from build123d import *

# Parameters (mm, degrees)
F0_R     = 12.7
F1_DEPTH = 152.4
F3_DEPTH = 127
F4_R     = 25.4
F5_SIZE  = 12.7


with BuildPart() as f1:
    # F0 (on Top) → F1 (new body)
    with BuildSketch(Plane.XY):
        with BuildLine():
            Line((127, 609.6), (0, 609.6))
            Line((0, 609.6), (0, 0))
            Line((0, 0), (115.211819, 0))
            ThreePointArc((115.211819, 0), (203.2, 76.2), (291.188181, 0))
            Line((291.188181, 0), (406.4, 0))
            Line((406.4, 0), (406.4, 609.6))
            Line((406.4, 609.6), (279.4, 609.6))
            ThreePointArc((279.4, 609.6), (203.2, 685.8), (127, 609.6))
        make_face()
        with Locations((203.2, 317.5)):
            Circle(F0_R, mode=Mode.SUBTRACT)
        with Locations((203.2, 628.65)):
            Circle(F0_R, mode=Mode.SUBTRACT)
    extrude(amount=F1_DEPTH)

    # F2 (on face) → F3 (cut)
    with BuildSketch(Plane(origin=(0, 0, 0), x_dir=(1, 0, 0), z_dir=(0, 0, -1))):
        with BuildLine():
            ThreePointArc((76.2, -107.95), (58.239488, -115.389488), (50.8, -133.35))
            Line((50.8, -133.35), (50.8, -533.4))
            ThreePointArc((50.8, -533.4), (58.239488, -551.360512), (76.2, -558.8))
            Line((76.2, -558.8), (330.2, -558.8))
            ThreePointArc((330.2, -558.8), (348.160512, -551.360512), (355.6, -533.4))
            Line((355.6, -533.4), (355.6, -133.35))
            ThreePointArc((355.6, -133.35), (348.160512, -115.389488), (330.2, -107.95))
            Line((330.2, -107.95), (76.2, -107.95))
        make_face()
    extrude(amount=-F3_DEPTH, mode=Mode.SUBTRACT)

    # F4
    f4_edges = [f1.edges().sort_by_distance(p)[0] for p in [
        (50.8, 333.375, 127),
    ]]
    fillet(f4_edges, radius=F4_R)

    # F5
    f5_edges = [f1.edges().sort_by_distance(p)[0] for p in [
        (406.4, 304.8, 152.4),
        (0, 304.8, 152.4),
    ]]
    chamfer(f5_edges, length=F5_SIZE)


solid = f1.part
Model file for the job. Use its own axes, mm. A direction names the side the tool comes from. Coordinates: 2 decimals unless noted, no trailing zeros. Write each loop counter-clockwise with the first axis right and the second up, starting at its lowest first coordinate (ties: lowest second). Pieces come first, ordered by that corner, then holes. Notation, with made-up numbers: (-31, -33.75) -> (3, -33.75) arc R28 cw to (3, 1.25) -> close; hole circle Ø6 at (4.25, -11). An arc over 180 degrees is marked (long way). One line per item, written item: value. Start each with the question number.
1) Which spindle directions (+Z, -Z, +X, -X, +Y, -Y) get a long thin tool onto all of the face, cutting with end or side? Do faces 4 (the face through (204.88, 685.78, 75.13)), 5 (the face through (348.36, 115.59, 50.09)), 6 (the face through (344, 609.6, 75)). Say none if no direction does.
2) Probe probe 1 along Y at (x, z) = (203.2, 103.5); probe 2 along Y at (x, z) = (203.2, 142); probe 3 along X at (y, z) = (283.5, 22.5). List the from-to ranges inside material, lowest first.
3) Slice it at D-D on x = 97.5. Write the cut outline in (y, z).
4) Slice it at A-A on y = 317.5. Write the cut outline in (x, z).
5) Slice it at B-B on z = 49.5. Write the cut outline in (x, y).
6) Flat gauge pins, fed straight in: pin 1 Ø3 at (x, y) = (299, 419) entering from -Z; pin 2 Ø23 at (x, y) = (203.2, 628.65) entering from +Z; pin 3 Ø10 at (x, y) = (111, 124.5) entering from -Z; pin 4 Ø3 at (x, y) = (96.5, 126) entering from -Z. Where does each tip first touch, or does it go through?
7) Pull direction X, two halves, no side cores. Call faces 1 (the face through (348, 0, 75)), 2 (the face through (6.4, 309.1, 146.1)), 3 (the face through (58.44, 115.19, 50.09)): +X half, -X half, draft (parallel to the pull), parting line (faces both ways), or undercut.
8) Slice it at C-C on x = 203.2. Write the cut outline in (y, z).
Answers follow:
1. face 4: +Z, -Z, +Y
1. face 5: -Z
1. face 6: +Z, -Z, +X, +Y
2. probe 1: 76.2 to 108.02, 558.73 to 615.95, 641.35 to 685.8
2. probe 2: 76.2 to 304.8, 330.2 to 615.95, 641.35 to 685.8
2. probe 3: 0 to 50.8, 355.6 to 406.4
3. outline: (0, 0) -> (107.95, 0) -> (107.95, 101.6) arc R25.4 cw to (133.35, 127) -> (533.4, 127) arc R25.4 cw to (558.8, 101.6) -> (558.8, 0) -> (609.6, 0) -> (609.6, 152.4) -> (0, 152.4) -> close
4. outline: (0, 0) -> (50.8, 0) -> (50.8, 101.6) arc R25.4 cw to (76.2, 127) -> (190.5, 127) -> (190.5, 152.4) -> (12.7, 152.4) -> (0, 139.7) -> close; (215.9, 127) -> (330.2, 127) arc R25.4 cw to (355.6, 101.6) -> (355.6, 0) -> (406.4, 0) -> (406.4, 139.7) -> (393.7, 152.4) -> (215.9, 152.4) -> close
5. outline: (0, 0) -> (115.21, 0) arc R88.9 cw to (291.19, 0) -> (406.4, 0) -> (406.4, 609.6) -> (279.4, 609.6) arc R76.2 ccw to (127, 609.6) -> (0, 609.6) -> close; hole (50.8, 133.35) arc R25.4 ccw to (76.2, 107.95) -> (330.2, 107.95) arc R25.4 ccw to (355.6, 133.35) -> (355.6, 533.4) arc R25.4 ccw to (330.2, 558.8) -> (76.2, 558.8) arc R25.4 ccw to (50.8, 533.4) -> close; hole circle Ø25.4 at (203.2, 628.65)
6. pin 1: z = 127
6. pin 2: through
6. pin 3: z = 122.89
6. pin 4: z = 125.41
7. face 1: draft
7. face 2: -X half
7. face 3: undercut
8. outline: (76.2, 0) -> (107.95, 0) -> (107.95, 101.6) arc R25.4 cw to (133.35, 127) -> (304.8, 127) -> (304.8, 152.4) -> (76.2, 152.4) -> close; (330.2, 127) -> (533.4, 127) arc R25.4 cw to (558.8, 101.6) -> (558.8, 0) -> (615.95, 0) -> (615.95, 152.4) -> (330.2, 152.4) -> close; (641.35, 0) -> (685.8, 0) -> (685.8, 152.4) -> (641.35, 152.4) -> close
